Check sheet for the drawn part. Datum: minimum x, y, z corner. Units: mm. A direction names the side the tool comes from. Round coordinates to 2 decimals unless told otherwise and drop trailing zeros. Write each loop counter-clockwise with the first axis right and the second up, starting at its lowest first coordinate (ties: lowest second). Pieces come first, ordered by that corner, then holes. Notation, with made-up numbers: M 39.25,69 L 85.25,69 A7 cw 85.25,81 Z; hole C -14,26.5 d6. An arc over 180 degrees is marked long. One line per item, written item: value.
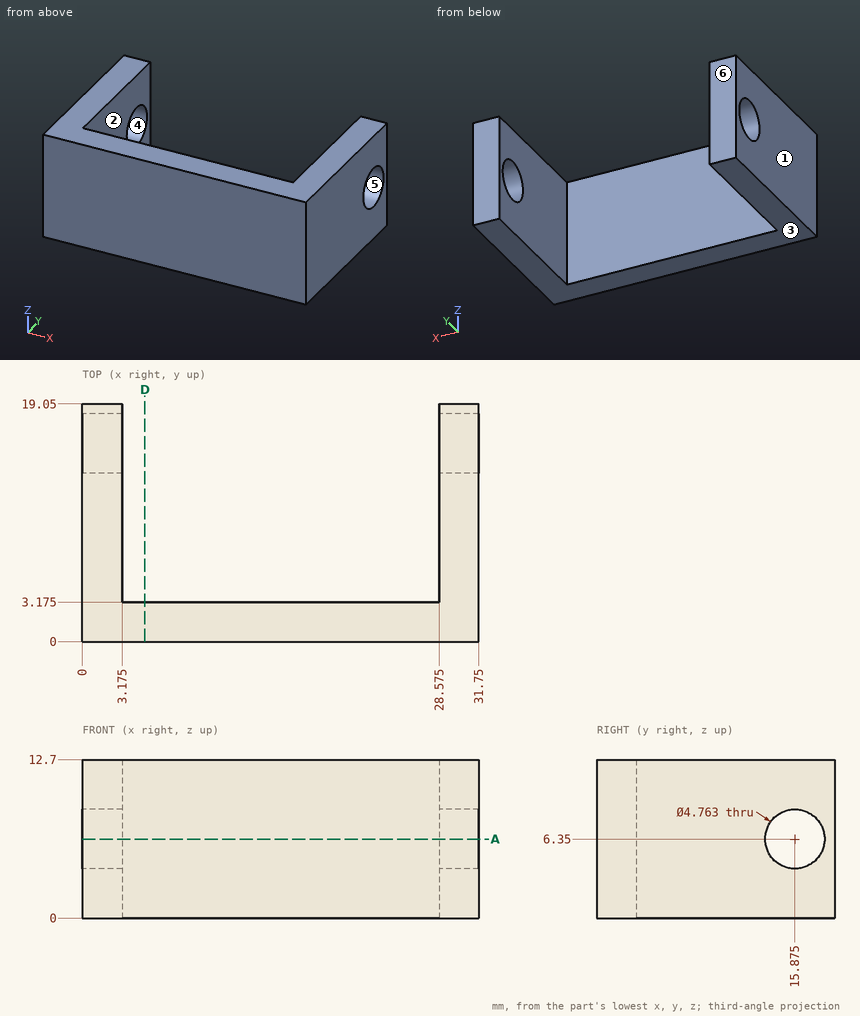
Q1. Scan lines: line 1 (Y direction, x = 30.9, z = 6.35); line 2 (Y direction, x = 9.5, z = 4.75) (1 decimal). Record each from-to range of solid material in increasing order. Write a range as [from, to].
Completed:
line 1: [0, 13.49], [18.26, 19.05]
line 2: [0, 3.2]
Q2. Draft check along Y on the marked faces 3, 4, 5 and 6. Enter one of: pulls with the +Y half, pulls with the -Y half, needs draft (parallel to the pull), parting line crosses it, or undercut.
Completed:
face 3: needs draft
face 4: undercut
face 5: undercut
face 6: pulls with the +Y half
Q3. Depth check by flat-ended pin: P1, Ø4, axis at x = 6, z = 9, coming from the +Y side (1 decimal); P2, Ø2, axis at y = 8.5, z = 6, coming from the -X side. Enter the tip coordinate at first touch or a pass-through.
Completed:
P1: y = 3.2
P2: x = 0
Q4. Sectioned sample at A-A on z = 6.35. State how many separate pieces and enclosed holes the cut face has, and give its area (3 significant figures).
Completed:
separate pieces: 3
enclosed holes: 0
area: 171 mm^2
Q5. Access from +Z, -Z, +X, -X, +Y, -Y to the whole of each face (thin tool, end or side, straight path). Record for the marked faces 1 and 2.
Completed:
face 1: +Z, -Z, -X, +Y, -Y
face 2: +Z, -Z, +Y
Q6. Sectioned sample at D-D on x = 5. Enter the section's corners in (y, z) (1 decimal).
Completed:
outline: M 0,0 L 3.2,0 L 3.2,12.7 L 0,12.7 Z
